```python
from build123d import *

# Parameters (mm, degrees)
EXTRUDE_1_DEPTH          = 35
SKETCH_2_R               = 10
SKETCH_2_R_2             = 15
CUT_EXTRUDE_1_DEPTH      = 1
CUT_EXTRUDE_1_DEPTH_BACK = 36
CUT_EXTRUDE_2_DEPTH      = 30
CUT_EXTRUDE_3_DEPTH      = 5
SKETCH_10_R              = 6
EXTRUDE_2_DEPTH          = 25
FILLET_1_R               = 10
HOLE_WIZARD_M4_1_D       = 3.3
HOLE_WIZARD_M4_1_DEPTH   = 11.5
HOLE_WIZARD_M4_1_TIP     = 0.991420021
HOLE_WIZARD_M4_2_D       = 3.3


with BuildPart() as part:
    # 스케치1 → 보스-돌출1 (new body)
    with BuildSketch(Plane(origin=(0, 0, 0), x_dir=(0, 0, -1), z_dir=(1, 0, 0))):
        with BuildLine():
            Line((-48.263014716, 12.710470067), (81.736985284, 12.710470067))
            ThreePointArc((81.736985284, 12.710470067), (116.736985284, -22.289529933), (81.736985284, -57.289529933))
            Line((81.736985284, -57.289529933), (-48.263014716, -57.289529933))
            ThreePointArc((-48.263014716, -57.289529933), (-83.263014716, -22.289529933), (-48.263014716, 12.710470067))
        make_face()
    extrude(amount=EXTRUDE_1_DEPTH)

    # 스케치2 → 컷-돌출1 (cut, two sides)
    with BuildSketch(Plane.ZY) as cut_extrude_1_sk:
        with Locations((23.263014716, -22.302890454)):
            Circle(SKETCH_2_R)
        with Locations((-81.736985284, -22.302890454)):
            Circle(SKETCH_2_R_2)
    extrude(amount=CUT_EXTRUDE_1_DEPTH, mode=Mode.SUBTRACT)
    extrude(cut_extrude_1_sk.sketch, amount=-CUT_EXTRUDE_1_DEPTH_BACK, mode=Mode.SUBTRACT)

    # 스케치3 → 컷-돌출2 (cut)
    with BuildSketch(Plane(origin=(35, 0, 0), x_dir=(0, 0, -1), z_dir=(1, 0, 0))):
        with BuildLine():
            Line((81.736985284, 7.710470067), (-48.263014716, 7.710470067))
            ThreePointArc((-48.263014716, 7.710470067), (-78.263014716, -22.289529933), (-48.263014716, -52.289529933))
            Line((-48.263014716, -52.289529933), (81.736985284, -52.289529933))
            ThreePointArc((81.736985284, -52.289529933), (111.736985284, -22.289529933), (81.736985284, 7.710470067))
        make_face()
    extrude(amount=-CUT_EXTRUDE_2_DEPTH, mode=Mode.SUBTRACT)

    # 스케치5 → 컷-돌출3 (cut)
    with BuildSketch(Plane(origin=(35, 0, 0), x_dir=(0, 0, -1), z_dir=(1, 0, 0))):
        with BuildLine():
            Line((-48.263014716, -54.289529933), (81.736985284, -54.289529933))
            ThreePointArc((81.736985284, -54.289529933), (113.736985284, -22.289529933), (81.736985284, 9.710470067))
            Line((81.736985284, 9.710470067), (-48.263014716, 9.710470067))
            ThreePointArc((-48.263014716, 9.710470067), (-80.263014716, -22.289529933), (-48.263014716, -54.289529933))
        make_face()
        with BuildLine():
            Line((-48.263014716, -52.289529933), (81.736985284, -52.289529933))
            ThreePointArc((81.736985284, -52.289529933), (111.736985284, -22.289529933), (81.736985284, 7.710470067))
            Line((81.736985284, 7.710470067), (-48.263014716, 7.710470067))
            ThreePointArc((-48.263014716, 7.710470067), (-78.263014716, -22.289529933), (-48.263014716, -52.289529933))
        make_face(mode=Mode.SUBTRACT)
    extrude(amount=-CUT_EXTRUDE_3_DEPTH, mode=Mode.SUBTRACT)

    # 스케치10 → 보스-돌출2 (add)
    with BuildSketch(Plane(origin=(5, 0, 0), x_dir=(0, 0, -1), z_dir=(1, 0, 0))):
        with Locations((16.736985284, 2.710470067)):
            Circle(SKETCH_10_R)
        with Locations((16.736985284, -47.289529933)):
            Circle(SKETCH_10_R)
    extrude(amount=EXTRUDE_2_DEPTH)

    # 필렛1
    fillet_1_edges = [part.edges().sort_by_distance(p)[0] for p in [
        (17.5, 7.710470067, -20.053610075),
        (17.5, 7.710470067, -13.420360494),
        (17.5, -52.289529933, -13.420360494),
        (17.5, -52.289529933, -20.053610075),
    ]]
    fillet(fillet_1_edges, radius=FILLET_1_R)

    # M4 나사 구멍1
    with Locations(Plane(origin=(30, 0, 0), x_dir=(0, 0, -1), z_dir=(1, 0, 0))):
        with Locations((16.736985284, 2.697109546), (16.736985284, -47.302890454)):
            Hole(HOLE_WIZARD_M4_1_D / 2, depth=HOLE_WIZARD_M4_1_DEPTH)
            with Locations((0, 0, -(HOLE_WIZARD_M4_1_DEPTH + HOLE_WIZARD_M4_1_TIP / 2))):  # 118° drill point
                Cone(0, HOLE_WIZARD_M4_1_D / 2, HOLE_WIZARD_M4_1_TIP, mode=Mode.SUBTRACT)

    # M4 나사 구멍2 (through all)
    with Locations(Plane(origin=(5, 0, 0), x_dir=(0, 0, -1), z_dir=(1, 0, 0))):
        with Locations((-33.869616434, -11.696288736), (-12.656412998, -11.696288736), (-12.656412998, -32.909492171), (-33.869616434, -32.909492171), (-53.263014716, -37.302890454), (-53.263014716, -22.302890454), (-53.263014716, -7.302890454), (81.736985284, -0.302890454), (101.736985284, -22.302890454), (81.736985284, -44.302890454), (31.736985284, -22.302890454)):
            Hole(HOLE_WIZARD_M4_2_D / 2)


solid = part.part
```
Geometry check sheet. Reference: the model listing, model coordinates, mm. A direction names the side the tool comes from. Give positions to 0.01 mm unless a question says otherwise; leave off trailing zeros. Write each loop counter-clockwise with the first axis right and the second up, starting at its lowest first coordinate (ties: lowest second). Pieces come first, ordered by that corner, then holes. Notation, with made-up numbers: (-35, 13) -> (16, 13) arc R17 cw to (16, 22) -> close; hole circle Ø4 at (-6, 13). An arc over 180 degrees is marked (long way). One line per question, with ' | ' between items.
Item 1: Scan lines: line 1 along Y through (x, z) = (8.5, 17); line 2 along Z through (x, y) = (19, 2.5); line 3 along Z through (x, y) = (4.5, -12). Record each from-to range of solid material in increasing order.
Determined:
line 1: -57.29 to -52.29, 7.71 to 12.71 | line 2: -106.44 to -98.63, -23.16 to -18.38, -15.1 to -10.32, 65.16 to 72.97 | line 3: -115.19 to -92.64, -70.84 to 11.03, 14.28 to 32.25, 35.49 to 81.72
Item 2: Draft check along Z on faces 3 (the cylindrical face through (2.465, -7.23, 51.615)), 4 (the cylindrical face through (32.53, -22.99, -113.73)). Enter one of: released by +Z, released by -Z, zero draft, split by the parting line, or undercut.
Determined:
face 3: undercut | face 4: undercut
Item 3: Access from +Z, -Z, +X, -X, +Y, -Y to the whole of each face (thin tool, end or side, straight path). Record for faces 1 (the cylindrical face through (2.465, -21.643, -96.722)), 2 (the flat face through (30, -3, -16)).
Determined:
face 1: +X, -X | face 2: +X
Item 4: Sectioned sample at B-B, the plane z = -89. Record the boundary of the cut face in (x, y), plus the area to 3 significant figures.
Determined:
outline: (0, -56.53) -> (35, -56.53) -> (35, -53.45) -> (30, -53.45) -> (30, -51.4) -> (5, -51.4) -> (5, -35.43) -> (0, -35.43) -> close; (0, -9.18) -> (5, -9.18) -> (5, 6.82) -> (30, 6.82) -> (30, 8.88) -> (35, 8.88) -> (35, 11.95) -> (0, 11.95) -> close | area: 498 mm^2
Item 5: Sectioned sample at D-D, the plane x = 21. Record the boundary of the cut face in (y, z), plus the area to 3 significant figures.
Determined:
outline: (-57.29, -81.74) arc R35 ccw to (12.71, -81.74) -> (12.71, 48.26) arc R35 ccw to (-57.29, 48.26) -> close; hole (-52.29, -81.74) arc R30 ccw to (7.71, -81.74) -> (7.71, -31.94) arc R10 ccw to (0.84, -22.44) arc R6 cw to (0.84, -11.04) arc R10 ccw to (7.71, -1.54) -> (7.71, 48.26) arc R30 ccw to (-52.29, 48.26) -> (-52.29, -1.54) arc R10 ccw to (-45.41, -11.04) arc R6 cw to (-45.41, -22.44) arc R10 ccw to (-52.29, -31.94) -> close; hole circle Ø3.3 at (-47.3, -16.74); hole circle Ø3.3 at (2.7, -16.74) | area: 2,600 mm^2
Item 6: Sectioned sample at A-A, the plane x = 32.5. Record the boundary of the cut face in (y, z), plus the area to 3 significant figures.
Determined:
outline: (-57.29, -81.74) arc R35 ccw to (12.71, -81.74) -> (12.71, 48.26) arc R35 ccw to (-57.29, 48.26) -> close; hole (-54.29, -81.74) arc R32 ccw to (9.71, -81.74) -> (9.71, 48.26) arc R32 ccw to (-54.29, 48.26) -> close | area: 1,410 mm^2
Item 7: Sectioned sample at C-C, the plane z = -39.5. Record the boundary of the cut face in (x, y), plus the area to 3 significant figures.
Determined:
outline: (0, -57.29) -> (35, -57.29) -> (35, -54.29) -> (30, -54.29) -> (30, -52.29) -> (5, -52.29) -> (5, 7.71) -> (30, 7.71) -> (30, 9.71) -> (35, 9.71) -> (35, 12.71) -> (0, 12.71) -> close | area: 630 mm^2
Item 8: Depth check by flat-ended pin: pin 1 (2 mm diameter, centred on y = -0.3, z = -81.74, fed in from -X); pin 2 (4 mm diameter, centred on x = 31, y = -15.5, fed in from -Z); pin 3 (4.5 mm diameter, centred on y = -22.3, z = -31.74, fed in from -X); pin 4 (18 mm diameter, centred on y = -13, z = -49, fed in from +X). Enter the tip coordinate at first touch or a pass-through.
Determined:
pin 1: through | pin 2: z = -116.41 | pin 3: x = 0 | pin 4: x = 5
